```python
from build123d import *

# Parameters (mm, degrees)
SALIENTE_EXTRUIR1_DEPTH = 5
CROQUIS2_R              = 1.25
CORTAR_EXTRUIR1_DEPTH   = 10
CORTAR_EXTRUIR2_DEPTH   = 22
CORTAR_EXTRUIR3_DEPTH   = 10
SALIENTE_EXTRUIR2_DEPTH = 5
CROQUIS7_R              = 1.25
CORTAR_EXTRUIR4_DEPTH   = 10
SALIENTE_EXTRUIR3_DEPTH = 5
CORTAR_EXTRUIR7_DEPTH   = 10


with BuildPart() as part:
    # Croquis1 → Saliente-Extruir1 (new body)
    with BuildSketch(Plane.XY):
        Polygon((94.71302301, -28.670259317), (124.784571975, -2.294096918), (121.487551675, 1.464846702), (33.971255169, 31.023525729), (29.162783478, 36.110627065), (4.554636507, 125.156882092), (0.987169784, 128.660192123), (-27.039310471, 100.120458339), (-30.489528096, 86.717422014), (-9.088639631, 9.652046375), (5.402210696, -5.678484568), (81.141270829, -31.381887447), align=None)
    extrude(amount=SALIENTE_EXTRUIR1_DEPTH)

    # Croquis2 → Cortar-Extruir1 (cut)
    with BuildSketch(Plane.XY.offset(5)):
        with Locations((27.933375513, 30.132453761)):
            Circle(CROQUIS2_R)
        with Locations((13.398800269, 16.393963215)):
            Circle(CROQUIS2_R)
    extrude(amount=-CORTAR_EXTRUIR1_DEPTH, mode=Mode.SUBTRACT)

    # Croquis3 → Cortar-Extruir2 (cut)
    with BuildSketch(Plane.XY.offset(5)):
        Polygon((32.261175329, -9.513472178), (57.513309445, -18.083234934), (55.906478928, -22.818010081), (30.654344812, -14.248247324), align=None)
        Polygon((101.439852365, -16.119261564), (111.46370202, -7.327207431), (114.76072232, -11.086151051), (104.736872665, -19.878205184), align=None)
        Polygon((-11.401313453, 36.666602778), (-18.536576351, 62.360943293), (-23.354265197, 61.023081499), (-16.219002299, 35.328740985), align=None)
        Polygon((-14.129683663, 106.130392902), (-4.787523578, 115.643637497), (-8.354990301, 119.146947529), (-17.697150386, 109.633702934), align=None)
    extrude(amount=-CORTAR_EXTRUIR2_DEPTH, mode=Mode.SUBTRACT)

    # Croquis4 → Cortar-Extruir3 (cut)
    with BuildSketch(Plane.XY.offset(5)):
        Polygon((-0.808419356, 84.479263676), (-5.626108202, 83.141401882), (0.082102116, 62.58592947), (4.899790963, 63.923791264), align=None)
        Polygon((55.750831206, 6.80326974), (54.144000689, 2.068494593), (74.345707981, -4.787315612), (75.952538498, -0.052540465), align=None)
    extrude(amount=-CORTAR_EXTRUIR3_DEPTH, mode=Mode.SUBTRACT)

    # Croquis5 → Saliente-Extruir2 (add)
    with BuildSketch(Plane.XY.offset(5)):
        Polygon((4.554636507, 125.156882092), (9.373993305, 126.488722946), (33.650829441, 38.641338728), (36.750129482, 35.362447971), (123.087510452, 6.201948338), (121.487551675, 1.464846702), (33.971255169, 31.023525729), (29.162783478, 36.110627065), align=None)
    extrude(amount=-SALIENTE_EXTRUIR2_DEPTH)

    # Croquis7 → Cortar-Extruir4 (cut)
    with BuildSketch(Plane(origin=(0, 0, 0), x_dir=(-1, 0, 0), z_dir=(0, 0, -1))):
        with Locations((-61.444669333, -22.057453024)):
            Circle(CROQUIS7_R)
        with Locations((-26.722984924, -10.274029234)):
            Circle(CROQUIS7_R)
        with Locations((12.472296082, 31.179983035)):
            Circle(CROQUIS7_R)
        with Locations((22.283282568, 66.509701242)):
            Circle(CROQUIS7_R)
    extrude(amount=-CORTAR_EXTRUIR4_DEPTH, mode=Mode.SUBTRACT)

    # Croquis8 → Saliente-Extruir3 (add)
    with BuildSketch(Plane(origin=(0, 0, 0), x_dir=(-1, 0, 0), z_dir=(0, 0, -1))):
        Polygon((-33.650829441, 38.641338728), (-9.373993305, 126.488722946), (-14.193350102, 127.8205638), (-38.138875404, 41.172050391), (-39.529003796, 39.701370213), (-124.68746923, 10.939049974), (-123.087510452, 6.201948338), (-36.750129482, 35.362447971), align=None)
    extrude(amount=-SALIENTE_EXTRUIR3_DEPTH)

    # Croquis9 → Cortar-Extruir7 (cut)
    with BuildSketch(Plane(origin=(0, 0, 0), x_dir=(-1, 0, 0), z_dir=(0, 0, -1))):
        Polygon((-119.772647147, -6.690123985), (-116.160686285, 13.818975774), (-124.68746923, 10.939049974), (-121.487551675, 1.464846702), (-124.784571975, -2.294096918), align=None)
        Polygon((3.683910258, 123.903569826), (-16.59066364, 119.145721565), (-14.193350102, 127.8205638), (-4.554636507, 125.156882092), (-0.987169784, 128.660192123), align=None)
    extrude(amount=-CORTAR_EXTRUIR7_DEPTH, mode=Mode.SUBTRACT)


solid = part.part
```
Work out the finished part from the listing and answer in its coordinate system (mm). A direction names the side the tool comes from. Round coordinates to 2 decimals unless told otherwise and drop trailing zeros. Loops run counter-clockwise (first coordinate to the right, second up) from the corner with the lowest first, then second, coordinate; pieces in that order, holes last. Notation, with made-up numbers: (11.25, 27) -> (37.25, 27) arc R17 cw to (37.25, 44) -> close; hole circle Ø6 at (-40, 22). An arc over 180 degrees is marked (long way). Write each question's results on one line, items separated by ' | '. Start each with the question number.
1. Find the intervals of material crossed by probe 1 along Y at (x, z) = (68, 0.45); probe 2 along X at (y, z) = (109.5, 2.5); probe 3 along Y at (x, z) = (-19.5, 0.8), in increasing order. Write a range as from..to.
2. Section A-A (x = 50.5) is taken. Determine the outline of the cut face in (y, z), plus the area to 3 significant figures.
3. Given pin 1 Ø2 at (y, z) = (65, 4) entering from -X; pin 2 Ø3 at (x, z) = (50, 3) entering from -Y; pin 3 Ø3 at (y, z) = (71.5, 2.5) entering from +X, each flat-ended and moving along its own axis, determine where each tip first touches the part or whether it passes through.
4. Section C-C (y = 23.5) is taken. Determine the outline of the cut face in (x, z).
5. A tool of negligible diameter and unlimited length cuts with its end or side. For faces 4 (the face through (117.992, 3.421, 2.465)), 5 (the face through (103.111, -18.025, 2.535)), 6 (the face through (-9.524, 110.82, 2.535)), 7 (the face through (-6.546, 117.371, 2.535)), from which of +Z, -Z, +X, -X, +Y, -Y can it reach the whole face along a straight path? Write none if from no direction.
6. Section B-B (z = 3.55) is taken. State how many separate pieces and enclosed holes the cut face has, plus the area to 3 significant figures.
7. For a pull along X with two mould halves and no side action, classify faces 1 (the face through (-15.94, 107.91, 2.54)), 2 (the face through (6.31, 121.56, 2.46)), 3 (the face through (-5.987, 121.559, 2.465)) as +X half, -X half, draft (parallel to the pull), parting line (faces both ways), or undercut.
Evaluation:
1) probe 1: y = -26.92..-2.63, 2.65..30.09 | probe 2: x = -17.83..-17.56, -10.82..19.26 | probe 3: y = 62.09..107.8
2) outline: (-15.7, 0) -> (36, 0) -> (36, 5) -> (-15.7, 5) -> close | area: 258 mm2
3) pin 1: stops at x = -24.74 | pin 2: stops at y = -16.04 | pin 3: stops at x = 30.17
4) outline: (-12.93, 0) -> (87.5, 0) -> (87.5, 5) -> (-12.93, 5) -> close
5) face 4: +Z, -Z, +X, +Y | face 5: +Z, -Z, +X | face 6: +Z, -Z | face 7: +Z, -Z, -X
6) separate pieces: 1 | enclosed holes: 8 | area: 9,800 mm2
7) face 1: undercut | face 2: +X half | face 3: -X half
